Design review of the part built by this model. Coordinates are the model's own, in mm. A direction names the side the tool comes from. Coordinates: 2 decimals unless noted, no trailing zeros. Loops run counter-clockwise (first coordinate to the right, second up) from the corner with the lowest first, then second, coordinate; pieces in that order, holes last. Notation, with made-up numbers: M 54,63 L 73,63 A36 ccw 73,100 Z; hole C 37.25,19 d11. An arc over 180 degrees is marked long. One line per item, written item: value.
```python
from build123d import *

# Parameters (mm, degrees)
BOSS_EXTRUDE1_DEPTH = 16
SKETCH4_R           = 2
CUT_EXTRUDE1_DEPTH  = 16
SKETCH6_W           = 2
SKETCH6_H           = 10
BOSS_EXTRUDE2_DEPTH = 12
CUT_EXTRUDE2_DEPTH  = 12
SKETCH8_R           = 2
CUT_EXTRUDE3_DEPTH  = 12
SKETCH9_R           = 4.5
CUT_EXTRUDE4_DEPTH  = 12


with BuildPart() as part:
    # Sketch1 → Boss-Extrude1 (new body)
    with BuildSketch(Plane(origin=(0, 0, 0), x_dir=(1, 0, 0), z_dir=(0, 1, 0))):
        Polygon((-17.922680412, 12.524914089), (-17.922680412, -17.975085911), (2.077319588, -17.975085911), (2.077319588, -15.975085911), (-15.922680412, -15.975085911), (-15.922680412, 12.524914089), align=None)
    extrude(amount=BOSS_EXTRUDE1_DEPTH)

    # Sketch4 → Cut-Extrude1 (cut)
    with BuildSketch(Plane.XY.offset(17.975085911)):
        with Locations((-12.922680412, 8)):
            Circle(SKETCH4_R)
        with Locations((-2.922680412, 8)):
            Circle(SKETCH4_R)
    extrude(amount=-CUT_EXTRUDE1_DEPTH, mode=Mode.SUBTRACT)

    # Sketch6 → Boss-Extrude2 (add)
    with BuildSketch(Plane.XZ):
        with Locations((-16.922680412, 2.725085911)):
            Rectangle(SKETCH6_W, SKETCH6_H)
    boss_extrude2 = extrude(amount=BOSS_EXTRUDE2_DEPTH)

    # Sketch7 → Cut-Extrude2 (cut)
    with BuildSketch(Plane(origin=(-15.922680412, 0, 0), x_dir=(0, 0, -1), z_dir=(1, 0, 0))):
        with BuildLine():
            Line((-11.171347401, -12.363043628), (4.929338565, -12.363043628))
            Line((4.929338565, -12.363043628), (4.929338565, -7))
            Line((4.929338565, -7), (2.274914089, -7))
            ThreePointArc((2.274914089, -7), (-2.725085911, -12), (-7.725085911, -7))
            Line((-7.725085911, -7), (-11.171347401, -7))
            Line((-11.171347401, -7), (-11.171347401, -12.363043628))
        make_face()
    cut_extrude2 = extrude(amount=-CUT_EXTRUDE2_DEPTH, mode=Mode.SUBTRACT)

    # Sketch8 → Cut-Extrude3 (cut)
    with BuildSketch(Plane(origin=(-15.922680412, 0, 0), x_dir=(0, 0, -1), z_dir=(1, 0, 0))):
        with Locations((-2.725085911, -9.5)):
            Circle(SKETCH8_R)
    cut_extrude3 = extrude(amount=-CUT_EXTRUDE3_DEPTH, mode=Mode.SUBTRACT)

    # Mirror1: Boss-Extrude2, Cut-Extrude2, Cut-Extrude3 across plane
    add(boss_extrude2.mirror(Plane(origin=(0, 8, 0), x_dir=(0, 0, 1), z_dir=(0, -1, 0))))
    add(cut_extrude2.mirror(Plane(origin=(0, 8, 0), x_dir=(0, 0, 1), z_dir=(0, -1, 0))), mode=Mode.SUBTRACT)
    add(cut_extrude3.mirror(Plane(origin=(0, 8, 0), x_dir=(0, 0, 1), z_dir=(0, -1, 0))), mode=Mode.SUBTRACT)

    # Sketch9 → Cut-Extrude4 (cut)
    with BuildSketch(Plane(origin=(-15.922680412, 0, 0), x_dir=(0, 0, -1), z_dir=(1, 0, 0))):
        with Locations((-9.475085911, 8)):
            Circle(SKETCH9_R)
    extrude(amount=-CUT_EXTRUDE4_DEPTH, mode=Mode.SUBTRACT)


solid = part.part
```
(1) Insertion check: pin 1 (1 mm diameter, centred on x = -16.5, y = -2, fed in from -Z); pin 2 (5 mm diameter, centred on x = -2.92, y = 8, fed in from +Z); pin 3 (0.6 mm diameter, centred on x = -17, z = -8.5, fed in from +Y); pin 4 (5 mm diameter, centred on y = 13.5, z = -2, fed in from +X). Each pin has a flat end and moves straight along its axis. Give the tip position at first contact, or say it passes through.
Reply:
pin 1: stops at z = -2.27
pin 2: stops at z = 17.98
pin 3: stops at y = 16
pin 4: stops at x = -15.92
(2) Mouldability with a two-part tool opening along Y and no side actions: class faces 4 (the cylindrical face through (-16.91, 8.2, 13.97)), 5 (the flat face through (2.077, 8, 17)), 6 (the flat face through (-17, 0, -7)), 7 (the flat face through (-11.7, 16, 16.2)) as released by +Y, released by -Y, zero draft, split by the parting line, or undercut.
Reply:
face 4: undercut
face 5: zero draft
face 6: released by -Y
face 7: released by +Y
(3) We need section C-C on y = -9. State the section outline as (x, z) points, then the cut area to 3 significant figures.
Reply:
outline: M -17.92,-1.86 L -15.92,-1.86 L -15.92,0.79 L -17.92,0.79 Z; M -17.92,4.66 L -15.92,4.66 L -15.92,7.31 L -17.92,7.31 Z
area: 10.6 mm2
(4) We need section D-D on x = -8.75. State the section outline as (y, z) points.
Reply:
outline: M 0,15.98 L 16,15.98 L 16,17.98 L 0,17.98 Z
(5) We need section B-B on x = -11.5. State the section outline as (y, z) points, then the cut area to 3 significant figures.
Reply:
outline: M 0,15.98 L 6.59,15.98 L 6.59,17.98 L 0,17.98 Z; M 9.41,15.98 L 16,15.98 L 16,17.98 L 9.41,17.98 Z
area: 26.4 mm2
(6) To check wall thickness, follow line 1 along X through (y, z) = (11, -1.5); line 2 along Z through (x, y) = (-11, 15); line 3 along Y through (x, z) = (-13.75, 17). State the ranges of each line that lie inside material, in increasing order. Write a range as [from, to].
Reply:
line 1: x = [-17.92, -15.92]
line 2: z = [15.98, 17.98]
line 3: y = [0, 6.18], [9.82, 16]
(7) We need section A-A on y = 8. State the section outline as (x, z) points, then the cut area to 3 significant figures.
Reply:
outline: M -17.92,-12.52 L -15.92,-12.52 L -15.92,4.98 L -17.92,4.98 Z; M -17.92,13.98 L -15.92,13.98 L -15.92,15.98 L -14.92,15.98 L -14.92,17.98 L -17.92,17.98 Z; M -10.92,15.98 L -4.92,15.98 L -4.92,17.98 L -10.92,17.98 Z; M -0.92,15.98 L 2.08,15.98 L 2.08,17.98 L -0.92,17.98 Z
area: 63.0 mm2
(8) Tool access review of faces 1 (the flat face through (-7, 8, 15.975)), 2 (the flat face through (-17, -3, 7.725)), 3 (the flat face through (-17, 19, -2.275)): name each direction out of +Z, -Z, +X, -X, +Y, -Y from which nothing blocks a thin tool from reaching the whole face with its end or side.
Reply:
face 1: -Z, +X, +Y, -Y
face 2: +Z, +X, -X, -Y
face 3: -Z, +X, -X, +Y
